Geometry: see drawing. Coordinates: mm, zero at the bounding-box minimum. A direction names the side the tool comes from. Coordinates: 2 decimals unless noted, no trailing zeros. Order: outer loops, then holes, each group sorted by start corner. A loop starts at its lowest first (then second) coordinate and runs counter-clockwise, first axis right, second up. Notation, with made-up numbers: (54, -28.5) -> (95, -28.5) arc R20 cw to (95, 1.5) -> close; hole circle Ø3 at (7, 31). An arc over 180 degrees is marked (long way). Use CSV: the item, a comma, the result in double quotes. Start each with the question number.
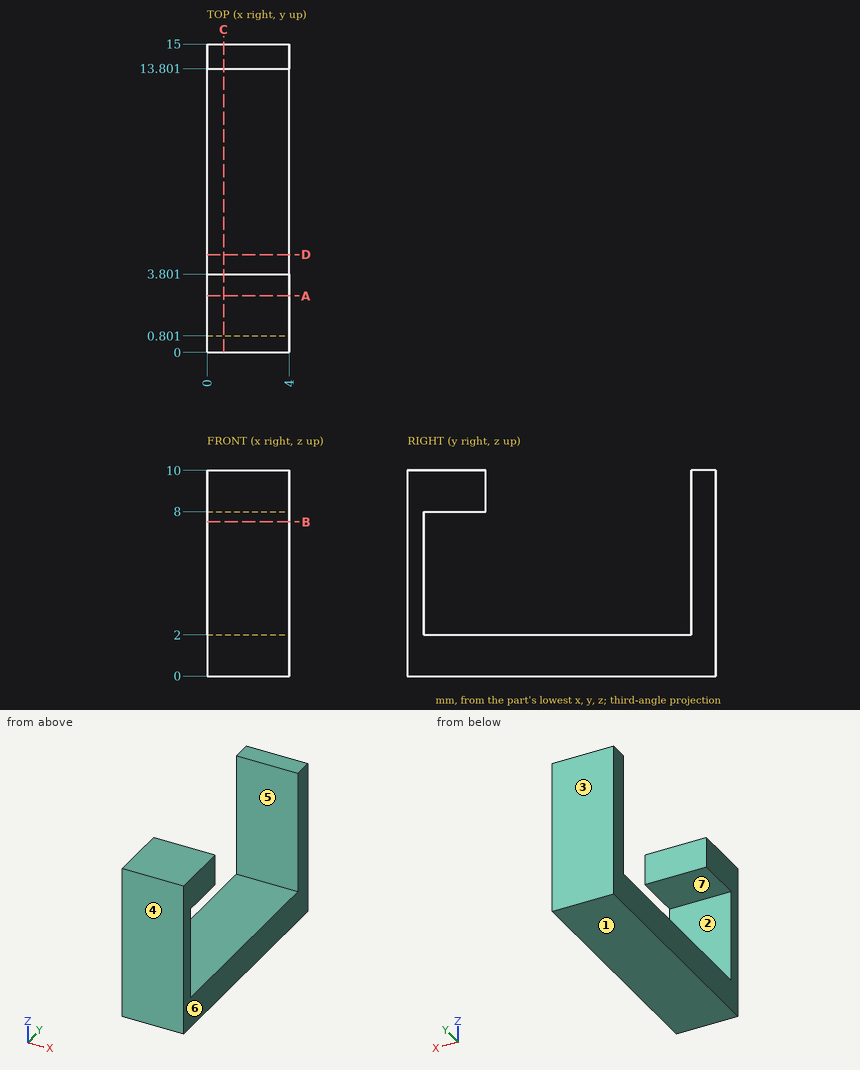
(1) Section D-D (y = 4.75). Return loops of the section in (x, z), then the cut area to 3 significant figures.
(2) Section A-A (y = 2.75). Return loops of the section in (x, z), then the cut area to 3 significant figures.
(3) Section B-B (z = 7.5). Return loops of the section in (x, y).
(4) Section C-C (x = 0.8). Return loops of the section in (y, z).
(5) Line query: line 1 (Y direction, x = 2.4, z = 2.75); line 2 (Y direction, x = 1.3, z = 8.5); line 3 (Z direction, x = 3.8, y = 3.5). Output: solid intervals per line, ascending. Write a range as from..to.
(6) Access query for the marked faces 5, 6 and 7. Directions: +Z, -Z, +X, -X, +Y, -Y. A direction counts if a zero-diameter tool reaches every point of the face in a straight line with its end or side. Return the directions, or none.
(7) Mould query, pull axis Y, two halves, no side actions, for the marked faces 1, 2, 3 and 4. Classes: pulls with the +Y half, pulls with the -Y half, needs draft (parallel to the pull), parting line crosses it, or undercut.
Check sheet entries:
1,outline,"(0, 0) -> (4, 0) -> (4, 2) -> (0, 2) -> close"
1,area,"8.00 mm^2"
2,outline,"(0, 0) -> (4, 0) -> (4, 2) -> (0, 2) -> close; (0, 8) -> (4, 8) -> (4, 10) -> (0, 10) -> close"
2,area,"16.0 mm^2"
3,outline,"(0, 0) -> (4, 0) -> (4, 0.8) -> (0, 0.8) -> close; (0, 13.8) -> (4, 13.8) -> (4, 15) -> (0, 15) -> close"
4,outline,"(0, 0) -> (15, 0) -> (15, 10) -> (13.8, 10) -> (13.8, 2) -> (0.8, 2) -> (0.8, 8) -> (3.8, 8) -> (3.8, 10) -> (0, 10) -> close"
5,line 1,"y = 0..0.8, 13.8..15"
5,line 2,"y = 0..3.8, 13.8..15"
5,line 3,"z = 0..2, 8..10"
6,face 5,"+Z, +X, -X"
6,face 6,"+Z, -Z, +X, +Y, -Y"
6,face 7,"+X, -X"
7,face 1,"needs draft"
7,face 2,"undercut"
7,face 3,"pulls with the +Y half"
7,face 4,"pulls with the -Y half"
